Can you work these out from the model? Positions are in its coordinate system, mm. Face numbers are marked on the shaded views. A direction names the side the tool comes from. Give positions to 0.01 mm unless a question says otherwise; leave off trailing zeros. Write each loop counter-clockwise with the first axis right and the second up, starting at its lowest first coordinate (ties: lowest second). Pieces come first, ordered by that corner, then holes. Notation, with made-up numbers: (19, 13.25) -> (32, 13.25) arc R37 cw to (32, 52.25) -> close; hole circle Ø11 at (20, 59.25). An arc over 180 degrees is marked (long way). One line per item, written item: value.
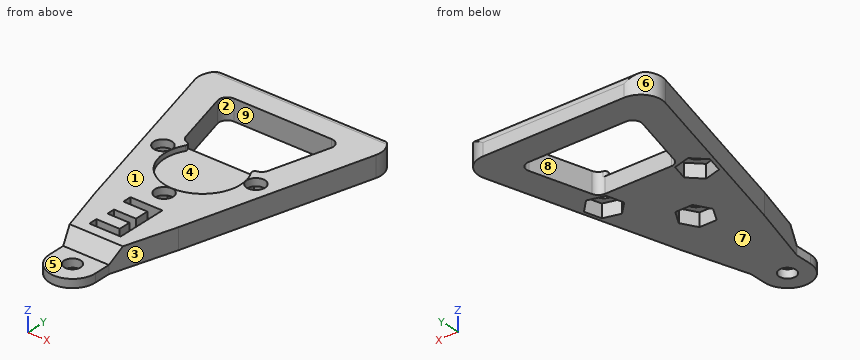
from build123d import *

# Parameters (mm, degrees)
BOSS_EXTRUDE1_DEPTH = 5
CUT_EXTRUDE1_REACH  = 36.673
SKETCH5_R           = 9.15
CUT_EXTRUDE3_DEPTH  = 1.2
CUT_EXTRUDE4_REACH  = 36.673
SKETCH6_R           = 2.2
CUT_EXTRUDE5_DEPTH  = 3.2
SKETCH8_W           = 20
SKETCH8_H           = 5
BOSS_EXTRUDE2_DEPTH = 15
SKETCH3_R           = 2
BOSS_EXTRUDE3_DEPTH = 5
CUT_EXTRUDE6_REACH  = 57.023
FILLET2_R           = 2
CUT_EXTRUDE7_DEPTH  = 3
CUT_EXTRUDE8_DEPTH  = 12.5
FILLET3_R           = 5
FILLET4_R           = 2
FILLET5_R           = 0.75


with BuildPart() as part:
    # Sketch1 → Boss-Extrude1 (new body)
    with BuildSketch(Plane.XY):
        Polygon((-23.5, 25), (23.5, 25), (10, -25), (-10, -25), align=None)
    extrude(amount=BOSS_EXTRUDE1_DEPTH)

    # Sketch2 → Cut-Extrude1 (cut, up to next)
    with BuildSketch(Plane.XY.offset(5), mode=Mode.PRIVATE) as cut_extrude1_sk1:
        Polygon((-9.499337961, 0), (9.499337961, 0), (14.359337961, 18), (-14.359337961, 18), align=None)
    cut_extrude1_tool1 = extrude(cut_extrude1_sk1.sketch, amount=-CUT_EXTRUDE1_REACH, mode=Mode.PRIVATE) & part.part
    add(cut_extrude1_tool1.solids().sort_by_distance((0, 9.611098, 5))[0], mode=Mode.SUBTRACT)

    # Sketch5 → Cut-Extrude3 (cut)
    with BuildSketch(Plane.XY.offset(5)):
        with Locations((0, -5.65)):
            Circle(SKETCH5_R)
    extrude(amount=-CUT_EXTRUDE3_DEPTH, mode=Mode.SUBTRACT)

    # Sketch6 → Cut-Extrude4 (cut, up to next)
    with BuildSketch(Plane.XY.offset(5), mode=Mode.PRIVATE) as cut_extrude4_sk1:
        with Locations((-11.197795542, -3.65)):
            Circle(SKETCH6_R)
    cut_extrude4_tool1 = extrude(cut_extrude4_sk1.sketch, amount=-CUT_EXTRUDE4_REACH, mode=Mode.PRIVATE) & part.part
    # Sketch6 → Cut-Extrude4 (cut, up to next)
    with BuildSketch(Plane.XY.offset(5), mode=Mode.PRIVATE) as cut_extrude4_sk2:
        with Locations((0, -17.025)):
            Circle(SKETCH6_R)
    cut_extrude4_tool2 = extrude(cut_extrude4_sk2.sketch, amount=-CUT_EXTRUDE4_REACH, mode=Mode.PRIVATE) & part.part
    # Sketch6 → Cut-Extrude4 (cut, up to next)
    with BuildSketch(Plane.XY.offset(5), mode=Mode.PRIVATE) as cut_extrude4_sk3:
        with Locations(Location((11.197795542, -3.65, 0), (0, 0, 180))):
            Circle(SKETCH6_R)
    cut_extrude4_tool3 = extrude(cut_extrude4_sk3.sketch, amount=-CUT_EXTRUDE4_REACH, mode=Mode.PRIVATE) & part.part
    add(cut_extrude4_tool1.solids().sort_by_distance((-11.197796, -3.65, 5))[0], mode=Mode.SUBTRACT)
    add(cut_extrude4_tool2.solids().sort_by_distance((0, -17.025, 5))[0], mode=Mode.SUBTRACT)
    add(cut_extrude4_tool3.solids().sort_by_distance((11.197796, -3.65, 5))[0], mode=Mode.SUBTRACT)

    # Sketch7 → Cut-Extrude5 (cut)
    with BuildSketch(Plane(origin=(0, 0, 0), x_dir=(-1, 0, 0), z_dir=(0, 0, -1))):
        Polygon((-7.208365159, -4.710791476), (-8.284407984, -0.72544768), (-12.273838367, 0.335343796), (-15.187225925, -2.589208524), (-14.1111831, -6.57455232), (-10.121752717, -7.635343796), align=None)
        Polygon((-4.128054425, -17.025), (-2.064027212, -20.6), (2.064027212, -20.6), (4.128054425, -17.025), (2.064027212, -13.45), (-2.064027212, -13.45), align=None)
        Polygon((10.121752717, -7.635343796), (14.1111831, -6.57455232), (15.187225925, -2.589208524), (12.273838367, 0.335343796), (8.284407984, -0.72544768), (7.208365159, -4.710791476), align=None)
    extrude(amount=-CUT_EXTRUDE5_DEPTH, mode=Mode.SUBTRACT)

    # Sketch8 → Boss-Extrude2 (add)
    with BuildSketch(Plane.XZ.offset(25)):
        with Locations((0, 2.5)):
            Rectangle(SKETCH8_W, SKETCH8_H)
    extrude(amount=BOSS_EXTRUDE2_DEPTH)

    # Sketch3 → Boss-Extrude3 (add)
    with BuildSketch(Plane.XY.offset(5)):
        with BuildLine():
            Line((-5.5, -44), (-5.5, -40))
            Line((-5.5, -40), (5.5, -40))
            Line((5.5, -40), (5.5, -44))
            ThreePointArc((5.5, -44), (0, -49.5), (-5.5, -44))
        make_face()
        with Locations((0, -44)):
            Circle(SKETCH3_R, mode=Mode.SUBTRACT)
    extrude(amount=-BOSS_EXTRUDE3_DEPTH)

    # Sketch9 → Cut-Extrude6 (cut, up to next)
    with BuildSketch(Plane(origin=(0, 0, 0), x_dir=(-1, 0, 0), z_dir=(0, 0, -1)), mode=Mode.PRIVATE) as cut_extrude6_sk1:
        Polygon((-10, -25), (-5.5, -40), (-10, -40), align=None)
    cut_extrude6_tool1 = extrude(cut_extrude6_sk1.sketch, amount=-CUT_EXTRUDE6_REACH, mode=Mode.PRIVATE) & part.part
    # Sketch9 → Cut-Extrude6 (cut, up to next)
    with BuildSketch(Plane(origin=(0, 0, 0), x_dir=(-1, 0, 0), z_dir=(0, 0, -1)), mode=Mode.PRIVATE) as cut_extrude6_sk2:
        Polygon((10, -25), (5.5, -40), (10, -40), align=None)
    cut_extrude6_tool2 = extrude(cut_extrude6_sk2.sketch, amount=-CUT_EXTRUDE6_REACH, mode=Mode.PRIVATE) & part.part
    add(cut_extrude6_tool1.solids().sort_by_distance((8.5, -35, 0))[0], mode=Mode.SUBTRACT)
    add(cut_extrude6_tool2.solids().sort_by_distance((-8.5, -35, 0))[0], mode=Mode.SUBTRACT)

    # Fillet2
    fillet2_edges = [part.edges().sort_by_distance(p)[0] for p in [
        (-9.499337961, 0, 2.5),
        (-14.359337961, 18, 2.5),
        (14.359337961, 18, 2.5),
        (9.499337961, 0, 2.5),
    ]]
    fillet(fillet2_edges, radius=FILLET2_R)

    # Sketch12 → Cut-Extrude7 (cut)
    with BuildSketch(Plane.XY.offset(5)):
        Polygon((3.812269091, -22.169612745), (3.812269091, -34.497542433), (-3.712571108, -34.497542433), (-3.712571108, -32.416203654), (1.891033295, -32.416203654), (1.891033295, -29.534349961), (-3.392365142, -29.534349961), (-3.392365142, -27.613114166), (1.891033295, -27.613114166), (1.891033295, -24.250951523), (-3.872674091, -24.250951523), (-3.872674091, -22.169612745), align=None)
    extrude(amount=-CUT_EXTRUDE7_DEPTH, mode=Mode.SUBTRACT)

    # Sketch13 → Cut-Extrude8 (cut, symmetric)
    with BuildSketch(Plane.ZY.offset(5.5)):
        Polygon((5, -37), (2, -40), (2, -51.866140446), (5, -51.866140446), align=None)
    extrude(amount=CUT_EXTRUDE8_DEPTH, both=True, mode=Mode.SUBTRACT)

    # Fillet3
    fillet3_edges = [part.edges().sort_by_distance(p)[0] for p in [
        (-23.5, 25, 2.5),
        (23.5, 25, 2.5),
    ]]
    fillet(fillet3_edges, radius=FILLET3_R)

    # Fillet4
    # the kernel refuses this fillet: 2 mm, written as the material it takes off along each edge
    with BuildSketch(Plane(origin=(-21.970955687, 25, 5), x_dir=(0, 0, -1), z_dir=(1, 0, 0))) as fillet4_piece_1:
        with BuildLine():
            CenterArc((FILLET4_R, -FILLET4_R), FILLET4_R, 90, 90)
            Line((0, -FILLET4_R), (0, 0))
            Line((0, 0), (FILLET4_R, 0))
        make_face()
    extrude(amount=43.941911373, mode=Mode.SUBTRACT)

    # Fillet5
    # the kernel refuses this fillet: 0.75 mm, written as the material it takes off along each edge
    with BuildSketch(Plane(origin=(-7.197221686, 0, 3.8), x_dir=(-0.999217435066786, 0.03955398157649034, 0), z_dir=(0, 0, 1))) as fillet5_piece_1:
        with BuildLine():
            CenterArc((1.339281213, 0.737984469), FILLET5_R, 152.162782465, 107.567464563)
            Line((0.676072834, 1.088205323), (0.609751996, 1.123227408))
            ThreePointArc((0.609751996, 1.123227408), (0.293398819, 0.571834806), (-0.060779257, 0.043941801))
            Line((-0.060779257, 0.043941801), (0.002966549, -0.074941308))
            ThreePointArc((0.002966549, -0.074941308), (0.772862133, -0.044465022), (1.192197913, -0.073798447))
            Line((1.192197913, -0.073798447), (1.205569122, 0))
        make_face()
    extrude(amount=4.402796923, mode=Mode.SUBTRACT)
    with BuildSketch(Plane(origin=(7.197221686, 0, 3.8), x_dir=(0.999217435066786, 0.039553981576491995, 0), z_dir=(0, 0, 1))) as fillet5_piece_2:
        with BuildLine():
            CenterArc((1.339281213, -0.737984469), FILLET5_R, 100.269752973, 107.567464563)
            Line((0.676072834, -1.088205323), (0.609751996, -1.123227408))
            ThreePointArc((0.609751996, -1.123227408), (0.293398819, -0.571834806), (-0.060779257, -0.043941801))
            Line((-0.060779257, -0.043941801), (0.002966549, 0.074941308))
            ThreePointArc((0.002966549, 0.074941308), (0.772862133, 0.044465022), (1.192197913, 0.073798447))
            Line((1.192197913, 0.073798447), (1.205569122, 0))
        make_face()
    extrude(amount=4.402796923, mode=Mode.SUBTRACT)


solid = part.part
1) If we section it at A-A (y = 9): Write out the boundary of the cut face in (x, z).
Answer list:
outline: (-19.18, 0) -> (-11.93, 0) -> (-11.93, 5) -> (-19.18, 5) -> close; (11.93, 0) -> (19.18, 0) -> (19.18, 5) -> (11.93, 5) -> close
2) We'd pull the mould along Y, two halves only. Please class the marked faces 6, 7, 8 and 9: released by +Y, released by -Y, zero draft, split by the parting line, or undercut.
Answer list:
face 6: split by the parting line
face 7: zero draft
face 8: undercut
face 9: undercut
3) Will these pins go through, and if not, where does the flat tip stop? pin 1 (3 mm diameter, centred on x = -1, y = -45, fed in from +Z); pin 2 (2.5 mm diameter, centred on x = -1.5, z = 2.5, fed in from -Y); pin 3 (3.5 mm diameter, centred on x = 1, y = -18.5, fed in from -Z); pin 4 (1.5 mm diameter, centred on x = -5.5, y = -39, fed in from -Z).
Answer list:
pin 1: stops at z = 2
pin 2: stops at y = -49.49
pin 3: stops at z = 3.2
pin 4: stops at z = 0
4) If we section it at C-C (y = -26.5): Write out the boundary of the cut face in (x, z), and give its area (3 significant figures).
Answer list:
outline: (-9.55, 0) -> (9.55, 0) -> (9.55, 5) -> (3.81, 5) -> (3.81, 2) -> (1.89, 2) -> (1.89, 5) -> (-9.55, 5) -> close
area: 89.7 mm^2
5) If we section it at B-B (y = -3.65): Write out the boundary of the cut face in (x, z), and give its area (3 significant figures).
Answer list:
outline: (-15.76, 0) -> (-14.9, 0) -> (-14.9, 3.2) -> (-13.4, 3.2) -> (-13.4, 5) -> (-15.76, 5) -> close; (-9, 3.2) -> (-7.49, 3.2) -> (-7.49, 0) -> (7.49, 0) -> (7.49, 3.2) -> (9, 3.2) -> (9, 5) -> (8.93, 5) -> (8.93, 3.8) -> (-8.93, 3.8) -> (-8.93, 5) -> (-9, 5) -> close; (13.4, 3.2) -> (14.9, 3.2) -> (14.9, 0) -> (15.76, 0) -> (15.76, 5) -> (13.4, 5) -> close
area: 73.0 mm^2
6) If we section it at D-D (y = -12): Write out the boundary of the cut face in (x, z).
Answer list:
outline: (-13.51, 0) -> (13.51, 0) -> (13.51, 5) -> (6.59, 5) -> (6.59, 3.8) -> (-6.59, 3.8) -> (-6.59, 5) -> (-13.51, 5) -> close
7) I need wall thicknesses on L1, parallel to Y at x = 0, z = 1.05; L2, parallel to Y at x = 4, z = 2.15; L3, parallel to X at y = -5, z = 2.2. Which ranges of each line are inside material? Lowest first, please.
Answer list:
L1: y = -49.5 to -46, -42 to -20.6, -13.45 to 0, 18 to 25
L2: y = -39.85 to -17.25, -16.8 to 0, 18 to 25
L3: x = -15.4 to -14.54, -7.5 to 7.5, 14.54 to 15.4
8) For the marked faces 1, 2, 3, 4 and 5, which set-ups out of +Z, -Z, +X, -X, +Y, -Y let a thin tool reach every point of the face, with its end or its side?
Answer list:
face 1: +Z, +X, -X, +Y, -Y
face 2: +Z, -Z
face 3: +Z, -Z, +X, -Y
face 4: +Z
face 5: +Z, +X, -X, -Y
